The drawing under review shows one solid part. Ordinate dimensions are in mm from its lowest x, y, z. Round coordinates to 2 decimals unless told otherwise and drop trailing zeros. Order: outer loops, then holes, each group sorted by start corner. A loop starts at its lowest first (then second) coordinate and runs counter-clockwise, first axis right, second up. Notation, with made-up numbers: M 18,65.25 L 30,65.25 A34 ccw 30,103.25 Z; hole C 51,-21 d6. An arc over 180 degrees is marked long. Use a Markdown table: item, result.
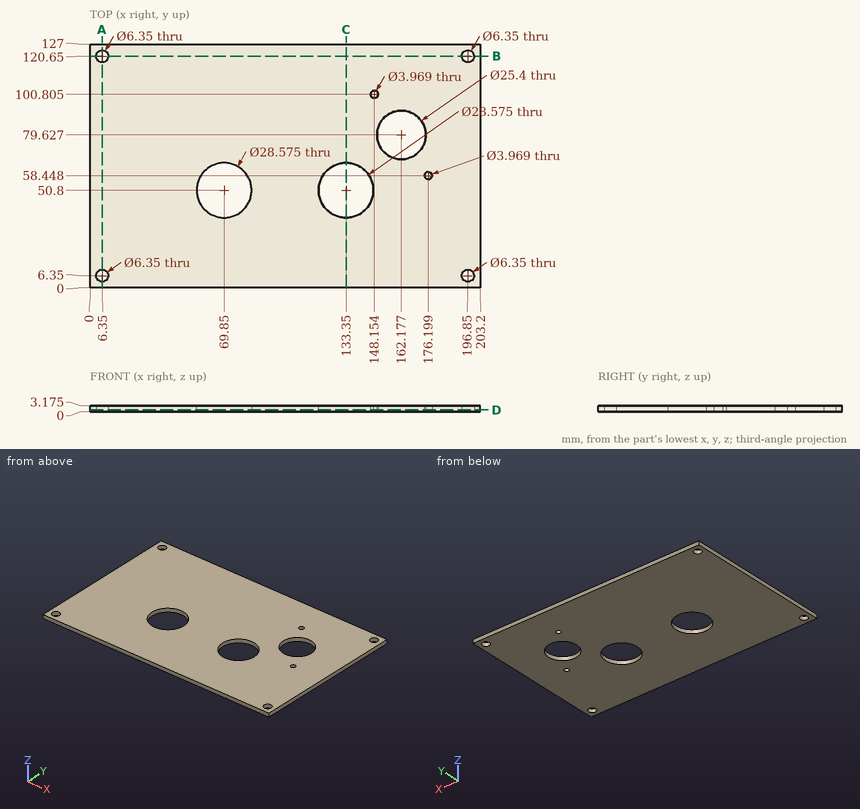
Q1. Add section A-A (x = 6.35). Write out the cut boundary in (y, z) (1 decimal), then the cut area to 3 significant figures.
Determined:
| item | result |
|---|---|
| outline | M 0,0 L 3.2,0 L 3.2,3.2 L 0,3.2 Z; M 9.5,0 L 117.5,0 L 117.5,3.2 L 9.5,3.2 Z; M 123.8,0 L 127,0 L 127,3.2 L 123.8,3.2 Z |
| area | 363 mm^2 |
Q2. Add section D-D (z = 1.05). Give the number of separate pieces and of enclosed holes in the cut face, then the cut area to 3 significant figures.
Determined:
| item | result |
|---|---|
| separate pieces | 1 |
| enclosed holes | 9 |
| area | 23,900 mm^2 |
Q3. Wall thickness on line 1 along X through (y, z) = (6.35, 0.9) (1 decimal); line 2 along Y through (x, z) = (196.85, 0.7) (1 decimal); line 3 along Y through (x, z) = (161.5, 2.9) (1 decimal): over which ranges is each line inside the solid? List them lowest first. Write a range as [from, to].
Determined:
| item | result |
|---|---|
| line 1 | x = [0, 3.2], [9.5, 193.7], [200, 203.2] |
| line 2 | y = [0, 3.2], [9.5, 117.5], [123.8, 127] |
| line 3 | y = [0, 66.9], [92.3, 127] |
Q4. Clearance check with flat-ended pins moving along their axes: pin 1 (8.5 mm diameter, centred on x = 6.35, y = 6.35, fed in from +Z) (3 decimals); pin 2 (2.5 mm diameter, centred on x = 176.199, y = 58.448, fed in from +Z). State where each tip first meets the part, or that it passes through.
Determined:
| item | result |
|---|---|
| pin 1 | stops at z = 3.175 |
| pin 2 | passes through |
Q5. Add section C-C (x = 133.35). Write out the cut boundary in (y, z) (1 decimal).
Determined:
| item | result |
|---|---|
| outline | M 0,0 L 36.5,0 L 36.5,3.2 L 0,3.2 Z; M 65.1,0 L 127,0 L 127,3.2 L 65.1,3.2 Z |
Q6. Add section B-B (y = 120.65). Write out the cut boundary in (x, z) (1 decimal).
Determined:
| item | result |
|---|---|
| outline | M 0,0 L 3.2,0 L 3.2,3.2 L 0,3.2 Z; M 9.5,0 L 193.7,0 L 193.7,3.2 L 9.5,3.2 Z; M 200,0 L 203.2,0 L 203.2,3.2 L 200,3.2 Z |
